Source: CAD feature listing. Evaluate the final solid. Frame: model axes, mm. Face numbers are marked on the shaded views. A direction names the side the tool comes from. Coordinates: 2 decimals unless noted, no trailing zeros. Loops run counter-clockwise (first coordinate to the right, second up) from the corner with the lowest first, then second, coordinate; pieces in that order, holes last. Notation, with made-up numbers: (9.5, 89) - (42.5, 89) arc R18 ccw to (42.5, 94) - close; hole circle Ø5 at (-3, 86.25). An arc over 180 degrees is marked (long way). Use one line per item in the form item = value. Start each with the question number.
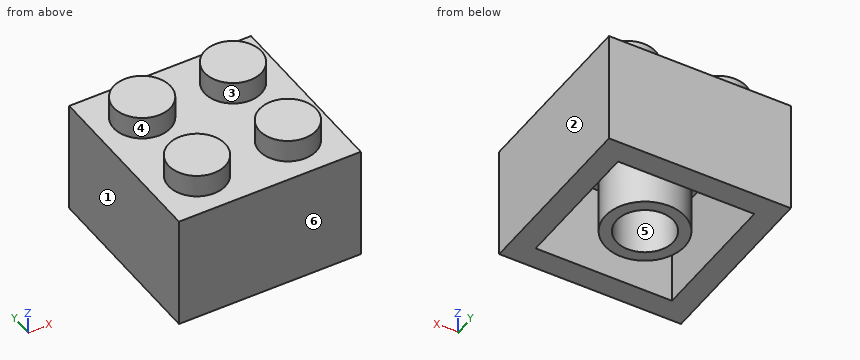
from build123d import *

# Parameters (mm, degrees)
F0_W     = 16
F0_H     = 10
F1_DEPTH = 16
F2_R     = 2.5
F3_DEPTH = 2
F5_W     = 12
F5_H     = 12
F5_R     = 3.5
F5_R_2   = 2.5
F6_DEPTH = 8
F7_R     = 1.25
F8_DEPTH = 9


with BuildPart() as f1:
    # F0 (on Front) → F1 (new body)
    with BuildSketch(Plane.XZ):
        with Locations((8, 5)):
            Rectangle(F0_W, F0_H)
    extrude(amount=F1_DEPTH)

    # F2 (on face) → F3 (join)
    with BuildSketch(Plane.XY.offset(10)):
        with Locations((4, -4)):
            Circle(F2_R)
        with Locations((12, -4)):
            Circle(F2_R)
        with Locations((4, -12)):
            Circle(F2_R)
        with Locations((12, -12)):
            Circle(F2_R)
    extrude(amount=F3_DEPTH)

    # F5 (on face) → F6 (cut)
    with BuildSketch(Plane(origin=(0, 0, 0), x_dir=(1, 0, 0), z_dir=(0, 0, -1))):
        with Locations((8, 8)):
            Rectangle(F5_W, F5_H)
        with Locations((8, 8)):
            Circle(F5_R, mode=Mode.SUBTRACT)
        with Locations((8, 8)):
            Circle(F5_R_2)
    extrude(amount=-F6_DEPTH, mode=Mode.SUBTRACT)

    # F7 (on face) → F8 (cut)
    with BuildSketch(Plane(origin=(0, 0, 0), x_dir=(1, 0, 0), z_dir=(0, 0, -1))):
        with Locations((12, 12)):
            Circle(F7_R)
        with Locations((4, 12)):
            Circle(F7_R)
        with Locations((4, 4)):
            Circle(F7_R)
        with Locations((12, 4)):
            Circle(F7_R)
    extrude(amount=-F8_DEPTH, mode=Mode.SUBTRACT)


solid = f1.part
(1) Cut plane A-A, the plane z = 7.75. Output: boundary loops of the cut face in (x, y), plus the area to 3 significant figures.
(2) Cut plane C-C, the plane z = 11.25. Output: boundary loops of the cut face in (x, y), plus the area to 3 significant figures.
(3) Access query for the marked faces 4, 5 and 6. Directions: +Z, -Z, +X, -X, +Y, -Y. A direction counts if a zero-diameter tool reaches every point of the face in a straight line with its end or side. Return the directions, or none.
(4) Material intervals for line 1 (X direction, y = -8, z = 2.5); line 2 (Y direction, x = 12, z = 8.3); line 3 (Y direction, x = 11.75, z = 5), sorted ascending.
(5) Mould query, pull axis X, two halves, no side actions, for the marked faces 1, 2 and 3. Classes: +X half, -X half, draft (parallel to the pull), parting line (faces both ways), or undercut.
(6) Cut plane D-D, the plane y = -4. Output: boundary loops of the cut face in (x, z), plus the area to 3 significant figures.
(7) Contact query for flat-ended pins moving along their axis: pin 1 (3 mm diameter, centred on x = 8, y = -8, fed in from +Z); pin 2 (1.2 mm diameter, centred on x = 4.5, y = -3.5, fed in from -Z); pin 3 (0.8 mm diameter, centred on x = 4, y = -12.5, fed in from -Z); pin 4 (3 mm diameter, centred on x = 8.5, y = -2.5, fed in from +Z). Output: stop coordinate, or through.
(8) Cut plane B-B, the plane x = 4. Output: boundary loops of the cut face in (y, z), plus the area to 3 significant figures.
Recorded:
q1.outline = (0, -16) - (16, -16) - (16, 0) - (0, 0) - close; circle Ø7 at (8, -8); hole (2, -14) - (14, -14) - (14, -2) - (2, -2) - close; hole circle Ø5 at (8, -8)
q1.area = 131 mm²
q2.outline = circle Ø5 at (4, -12); circle Ø5 at (4, -4); circle Ø5 at (12, -12); circle Ø5 at (12, -4)
q2.area = 78.5 mm²
q3.face_4 = +Z
q3.face_5 = -Z
q3.face_6 = +Z, -Z, +X, -X, -Y
q4.line_1 = 0 to 2, 4.5 to 5.5, 10.5 to 11.5, 14 to 16
q4.line_2 = -16 to -13.25, -10.75 to -5.25, -2.75 to 0
q4.line_3 = -16 to -14, -2 to 0
q5.face_1 = -X half
q5.face_2 = +X half
q5.face_3 = undercut
q6.outline = (0, 0) - (2, 0) - (2, 8) - (2.75, 8) - (2.75, 9) - (5.25, 9) - (5.25, 8) - (10.75, 8) - (10.75, 9) - (13.25, 9) - (13.25, 8) - (14, 8) - (14, 0) - (16, 0) - (16, 10) - (14.5, 10) - (14.5, 12) - (9.5, 12) - (9.5, 10) - (6.5, 10) - (6.5, 12) - (1.5, 12) - (1.5, 10) - (0, 10) - close
q6.area = 79.0 mm²
q7.pin_1 = 10
q7.pin_2 = 8
q7.pin_3 = 9
q7.pin_4 = 12
q8.outline = (-16, 0) - (-14, 0) - (-14, 8) - (-13.25, 8) - (-13.25, 9) - (-10.75, 9) - (-10.75, 8) - (-5.25, 8) - (-5.25, 9) - (-2.75, 9) - (-2.75, 8) - (-2, 8) - (-2, 0) - (0, 0) - (0, 10) - (-1.5, 10) - (-1.5, 12) - (-6.5, 12) - (-6.5, 10) - (-9.5, 10) - (-9.5, 12) - (-14.5, 12) - (-14.5, 10) - (-16, 10) - close
q8.area = 79.0 mm²
